Design review of the part built by this model. Coordinates are the model's own, in mm. Face numbers are marked on the shaded views. A direction names the side the tool comes from. Give positions to 0.01 mm unless a question says otherwise; leave off trailing zeros. Write each loop counter-clockwise with the first axis right and the second up, starting at its lowest first coordinate (ties: lowest second). Pieces come first, ordered by that corner, then holes. Notation, with made-up numbers: (-34, 28) - (-25, 28) arc R20 ccw to (-25, 40) - close; hole circle Ø7 at (-15.75, 46). An arc over 180 degrees is marked (long way). Write each question's results on one line, items separated by ' | '. Start each with the question number.
from build123d import *

# Parameters (mm, degrees)
SKETCH1_R      = 2.5
EXTRUDE1_DEPTH = 13
EXTRUDE2_DEPTH = 8
EXTRUDE3_START = 12
EXTRUDE3_DEPTH = 12
FILLET1_R      = 10
FILLET2_R      = 10
SKETCH4_R      = 2.5
EXTRUDE4_DEPTH = 112.725198761


with BuildPart() as part:
    # Sketch1 → Extrude1 (new body)
    with BuildSketch(Plane.XY):
        with BuildLine():
            Line((-9, 56.394324189), (-9, -99.519675811))
            ThreePointArc((-9, -99.519675811), (0, -108.519675811), (9, -99.519675811))
            Line((9, -99.519675811), (9, 56.394324189))
            ThreePointArc((9, 56.394324189), (0, 65.394324189), (-9, 56.394324189))
        make_face()
        with Locations(Location((0, 56.394324189, 0), (0, 0, 180))):
            Circle(SKETCH1_R, mode=Mode.SUBTRACT)
        with Locations(Location((0, -99.519675811, 0), (0, 0, 180))):
            Circle(SKETCH1_R, mode=Mode.SUBTRACT)
    extrude(amount=EXTRUDE1_DEPTH)

    # Sketch2 → Extrude2 (cut)
    with BuildSketch(Plane.XY.offset(13)):
        with BuildLine():
            Line((-5, -4.519675811), (-5, -84.519675811))
            ThreePointArc((-5, -84.519675811), (0, -89.519675811), (5, -84.519675811))
            Line((5, -84.519675811), (5, -4.519675811))
            ThreePointArc((5, -4.519675811), (0, 0.480324189), (-5, -4.519675811))
        make_face()
    extrude(amount=-EXTRUDE2_DEPTH, mode=Mode.SUBTRACT)

    # Sketch3 → Extrude3 (add)
    with BuildSketch(Plane(origin=(0, 0, 0), x_dir=(-1, 0, 0), z_dir=(0, 0, -1)).offset(EXTRUDE3_START)):
        with BuildLine():
            Line((-9, 56.394324189), (-9, 24.585637313))
            Line((-9, 24.585637313), (9, 24.585637313))
            Line((9, 24.585637313), (9, 56.394324189))
            ThreePointArc((9, 56.394324189), (0, 65.394324189), (-9, 56.394324189))
        make_face()
    extrude(amount=-EXTRUDE3_DEPTH)

    # Fillet1
    fillet1_edges = [part.edges().sort_by_distance(p)[0] for p in [
        (9, 24.585637313, -6),
    ]]
    fillet(fillet1_edges, radius=FILLET1_R)

    # Fillet2
    # the kernel refuses this fillet: 10 mm, written as the material it takes off along each edge
    with BuildSketch(Plane(origin=(-9, 24.585637313, -36.494897428), x_dir=(0, 1, 0), z_dir=(0, 0, 1))) as fillet2_piece_1:
        with BuildLine():
            CenterArc((9.797958971, -10), FILLET2_R, 90, 78.463040967)
            Line((0, -8), (-0.195959179, -7.96))
            ThreePointArc((-0.195959179, -7.96), (-0.2, -4), (-0.2, 0))
            Line((-0.2, 0), (0, 0.2))
            Line((0, 0.2), (9.797958971, 0.2))
            Line((9.797958971, 0.2), (9.797958971, 0))
        make_face()
    extrude(amount=36.494897428, mode=Mode.SUBTRACT)

    # Sketch4 → Extrude4 (cut, through all)
    with BuildSketch(Plane.XY.offset(13)):
        with Locations(Location((0, 56.394324189, 0), (0, 0, 180))):
            Circle(SKETCH4_R)
    extrude(amount=-EXTRUDE4_DEPTH, mode=Mode.SUBTRACT)


solid = part.part
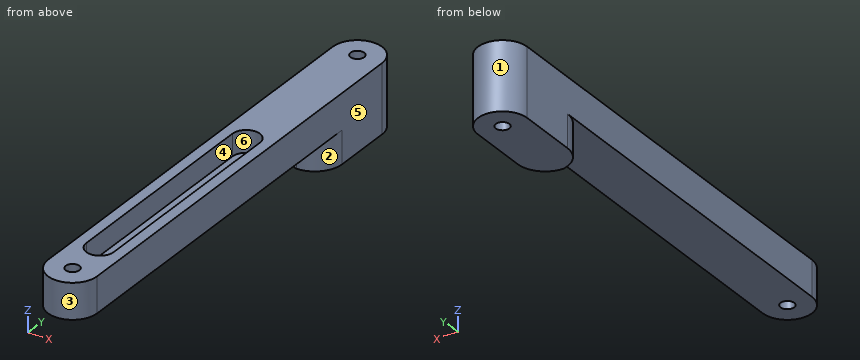
Q1. Add section C-C on y = 4. State the section outline as (x, z) points.
Q2. Add section B-B on y = -82. State the section outline as (x, z) points.
Q3. For line 1 along Y through (x, z) = (0, 4); line 2 along Y through (x, z) = (0, 8.5); line 3 along Z through (x, y) = (-6.5, 14.5), list the stretches that pass through material, from the lowest coordinate up. Write a range as [from, to].
Q4. Add section A-A on z = 2. State the section outline as (x, y) points.
Q5. Insertion check: P1, Ø3, axis at x = 3.5, z = 4.5, coming from the -Y side; P2, Ø8, axis at x = 0, y = 56.39, coming from the +Z side; P3, Ø3, axis at x = 1, y = -37, coming from the +Z side; P4, Ø5, axis at y = 16.5, z = -3.5, coming from the -X side. Each pin has a flat end and moves straight along its axis. Give the tip position at first contact, or say it passes through.
Q6. The part is to be moulded in two halves that separate along Y. For the marked faces 3, 4, 5 and 6, say which applies: +Y half, -Y half, draft (parallel to the pull), parting line (faces both ways), or undercut.
Q7. Machinability: for the marked faces 1 and 2, which of the approach directions +Z, -Z, +X, -X, +Y, -Y give a long, thin tool a straight path to every point of the face, cutting with its end or side? Answer none if there is none.
Result:
1) outline: (-9, 0) - (9, 0) - (9, 13) - (-9, 13) - close
2) outline: (-9, 0) - (9, 0) - (9, 13) - (5, 13) - (5, 5) - (-5, 5) - (-5, 13) - (-9, 13) - close
3) line 1: y = [-108.52, -102.02], [-97.02, 53.89], [58.89, 65.39] | line 2: y = [-108.52, -102.02], [-97.02, -89.52], [0.48, 53.89], [58.89, 65.39] | line 3: z = [0, 13]
4) outline: (-9, -99.52) arc R9 ccw to (9, -99.52) - (9, 56.39) arc R9 ccw to (-9, 56.39) - close; hole circle Ø5 at (0, -99.52); hole circle Ø5 at (0, 56.39)
5) P1: stops at y = -108.29 | P2: stops at z = 13 | P3: stops at z = 5 | P4: passes through
6) face 3: -Y half | face 4: undercut | face 5: draft | face 6: undercut
7) face 1: +Z, -Z, +Y | face 2: -Z, +X, -Y
